```python
from build123d import *

# Parameters (mm, degrees)
SKETCH2_R           = 4.1
BOSS_EXTRUDE1_DEPTH = 9.1
SKETCH3_R           = 3.1725
BOSS_EXTRUDE2_DEPTH = 14.7
CUT_EXTRUDE1_START  = -11
CUT_EXTRUDE1_DEPTH  = 11


with BuildPart() as part:
    # Sketch2 → Boss-Extrude1 (new body)
    with BuildSketch(Plane.XY):
        Circle(SKETCH2_R)
    extrude(amount=BOSS_EXTRUDE1_DEPTH)

    # Sketch3 → Boss-Extrude2 (add)
    with BuildSketch(Plane(origin=(0, 0, 0), x_dir=(-1, 0, 0), z_dir=(0, 0, -1))):
        Circle(SKETCH3_R)
    extrude(amount=BOSS_EXTRUDE2_DEPTH)

    # Sketch4 → Cut-Extrude1 (cut)
    with BuildSketch(Plane(origin=(0, 0, -14.7), x_dir=(-1, 0, 0), z_dir=(0, 0, -1)).offset(CUT_EXTRUDE1_START)):
        with BuildLine():
            Line((-2.737651106, 1.603129026), (2.737651106, 1.603129026))
            ThreePointArc((2.737651106, 1.603129026), (0, 3.1725), (-2.737651106, 1.603129026))
        make_face()
    extrude(amount=CUT_EXTRUDE1_DEPTH, mode=Mode.SUBTRACT)


solid = part.part
```
Here's how the part is built. I have some questions about the finished solid (model axes, mm). A direction names the side the tool comes from. Round coordinates to 2 decimals unless told otherwise and drop trailing zeros. Write each loop counter-clockwise with the first axis right and the second up, starting at its lowest first coordinate (ties: lowest second). Pieces come first, ordered by that corner, then holes. Notation, with made-up numbers: M 18,-36.5 L 73,-36.5 A7 cw 73,-27.5 Z; hole C -37,12.5 d10. An arc over 180 degrees is marked long. Answer as CSV lines item,"result". Start each with the question number.
1. Suppose I cut it at C-C on z = 2.25. Write out the boundary of the cut face in (x, y), then the cut area to 3 significant figures.
2. Suppose I cut it at D-D on y = 1. Write out the boundary of the cut face in (x, z), then the cut area to 3 significant figures.
3. Suppose I cut it at B-B on y = 0. Write out the boundary of the cut face in (x, z).
4. On a 3-axis mill with a long thin cutter (end or side, diameter ignored), from which of +Z, -Z, +X, -X, +Y, -Y can I reach the whole of each face in a straight line? I mean faces 1 (the cylindrical face through (0.688, -3.097, -7.247)), 2 (the flat face through (0, 2, -3.7)), 3 (the flat face through (0, -1, -14.7)). Say none if no direction works.
5. I'm going to push flat-ended pins straight in: pin 1 Ø1.5 at (y, z) = (2.5, -3.5) entering from -X; pin 2 Ø2.5 at (x, z) = (0.5, -7) entering from +Y; pin 3 Ø1.7 at (x, y) = (0, 2.5) entering from -Z. Where does each tip first touch, or does it pass through?
6. I need wall thicknesses on probe 1 along Z at (x, y) = (0.75, 3.5); probe 2 along Z at (x, y) = (-1.25, 2.5); probe 3 along X at (y, z) = (0.75, 5.5). Which ranges of each line are inside material? Lowest first, please.
7. Suppose I cut it at A-A on x = 0. Write out the boundary of the cut face in (y, z).
Check result:
1,outline,"C 0,0 d8.2"
1,area,"52.8 mm2"
2,outline,"M -3.98,0 L -3.01,0 L -3.01,-14.7 L 3.01,-14.7 L 3.01,0 L 3.98,0 L 3.98,9.1 L -3.98,9.1 Z"
2,area,"161 mm2"
3,outline,"M -4.1,0 L -3.17,0 L -3.17,-14.7 L 3.17,-14.7 L 3.17,0 L 4.1,0 L 4.1,9.1 L -4.1,9.1 Z"
4,face 1,"-Z"
4,face 2,"-Z, +X, -X, +Y"
4,face 3,"-Z, +X, -X, +Y, -Y"
5,pin 1,"stops at x = -2.65"
5,pin 2,"stops at y = 1.6"
5,pin 3,"stops at z = -3.7"
6,probe 1,"z = 0 to 9.1"
6,probe 2,"z = -3.7 to 9.1"
6,probe 3,"x = -4.03 to 4.03"
7,outline,"M -4.1,0 L -3.17,0 L -3.17,-14.7 L 1.6,-14.7 L 1.6,-3.7 L 3.17,-3.7 L 3.17,0 L 4.1,0 L 4.1,9.1 L -4.1,9.1 Z"
